```python
from build123d import *

# Parameters (mm, degrees)
BOSS_EXTRUDE1_DEPTH        = 20
BOSS_EXTRUDE2_DEPTH        = 20
FILLET1_R                  = 20
FILLET2_R                  = 25
F_0_2_0_2_DIAMETER_HOLE1_D = 0.2


with BuildPart() as part:
    # Sketch1 → Boss-Extrude1 (new body)
    with BuildSketch(Plane(origin=(0, 0, 0), x_dir=(1, 0, 0), z_dir=(0, 1, 0))):
        Polygon((0, 0), (0, 35), (150, 35), (150, -40), align=None)
    extrude(amount=BOSS_EXTRUDE1_DEPTH)

    # Sketch3 → Boss-Extrude2 (add)
    with BuildSketch(Plane(origin=(0, 0, -35), x_dir=(-1, 0, 0), z_dir=(0, 0, -1))):
        Polygon((-150, 0), (-150, 60), (-50, 80), (-50, 0), align=None)
    extrude(amount=-BOSS_EXTRUDE2_DEPTH)

    # Fillet1
    fillet1_edges = [part.edges().sort_by_distance(p)[0] for p in [
        (0, 10, 0),
    ]]
    fillet(fillet1_edges, radius=FILLET1_R)

    # Fillet2
    fillet2_edges = [part.edges().sort_by_distance(p)[0] for p in [
        (50, 80, -25),
        (150, 10, 40),
    ]]
    fillet(fillet2_edges, radius=FILLET2_R)

    # Ø0.2 (0.2) Diameter Hole1 (through all)
    with Locations(Plane(origin=(21.699653265, 20, -10.140884984), x_dir=(0, 0, 1), z_dir=(0, 1, 0))):
        with Locations((0, 0), (18.585454109, 104.917886097)):
            Hole(F_0_2_0_2_DIAMETER_HOLE1_D / 2)


solid = part.part
```
Input: part model. Units: mm. Frame: model coordinates. A direction names the side the tool comes from. Round coordinates to 2 decimals unless told otherwise and drop trailing zeros. Order: outer loops, then holes, each group sorted by start corner. A loop starts at its lowest first (then second) coordinate and runs counter-clockwise, first axis right, second up. Notation, with made-up numbers: (61, 66) - (96, 66) arc R14 ccw to (96, 93) - close; hole circle Ø9 at (-9, 23.25). An arc over 180 degrees is marked (long way). Answer in a Markdown table with one row per item.
Item 1: Reachability of faces 1 (the flat face through (99, 42, -15)), 2 (the cylindrical face through (4.25, 10.14, -3.04)), 3 (the flat face through (50, 35, -25)) from +Z, -Z, +X, -X, +Y, -Y: full face, straight path, thin tool, end or side. Return the list, or none.
Model answer:
| item | result |
|---|---|
| face 1 | +Z, +X, -X, +Y |
| face 2 | +Z, -X, +Y, -Y |
| face 3 | +Z, -Z, -X, +Y |
Item 2: Line query: line 1 (Z direction, x = 97, y = 23); line 2 (Y direction, x = 92, z = -6); line 3 (Z direction, x = 118.5, y = 11). Output: solid intervals per line, ascending.
Model answer:
| item | result |
|---|---|
| line 1 | z = -35 to -15 |
| line 2 | y = 0 to 20 |
| line 3 | z = -35 to 31.6 |
Item 3: Section query B-B (x = 105). Return the cut outline in (y, z), then the cut area to 3 significant figures.
Model answer:
| item | result |
|---|---|
| outline | (0, -35) - (69, -35) - (69, -15) - (20, -15) - (20, 28) - (0, 28) - close |
| area | 2,240 mm² |
Item 4: Pin query (flat end, axial travel): pin 1 (1 mm diameter, centred on x = 67.5, z = 10, fed in from +Y); pin 2 (10 mm diameter, centred on y = 38.5, z = -20, fed in from -X); pin 3 (3 mm diameter, centred on x = 67, y = 62.5, fed in from +Z). Return the tip coordinate at first contact, or that it passes through.
Model answer:
| item | result |
|---|---|
| pin 1 | stops at y = 20 |
| pin 2 | stops at x = 50 |
| pin 3 | stops at z = -15 |
Item 5: Section query D-D (y = 31.5). Return the cut outline in (x, z), then the cut area to 3 significant figures.
Model answer:
| item | result |
|---|---|
| outline | (50, -35) - (150, -35) - (150, -15) - (50, -15) - close |
| area | 2,000 mm² |
Item 6: Section query A-A (z = -27). Return the cut outline in (x, y), then the cut area to 3 significant figures.
Model answer:
| item | result |
|---|---|
| outline | (0, 0) - (150, 0) - (150, 60) - (79.9, 74.02) arc R25 ccw to (50, 49.5) - (50, 20) - (0, 20) - close |
| area | 7,790 mm² |
Item 7: Section query C-C (y = 10.5). Return the cut outline in (x, z).
Model answer:
| item | result |
|---|---|
| outline | (0, -35) - (150, -35) - (150, 7.46) arc R25 ccw to (118.56, 31.62) - (14.85, 3.96) arc R20 ccw to (0, -15.37) - close; hole circle Ø0.2 at (21.7, -10.14); hole circle Ø0.2 at (126.62, 8.44) |
